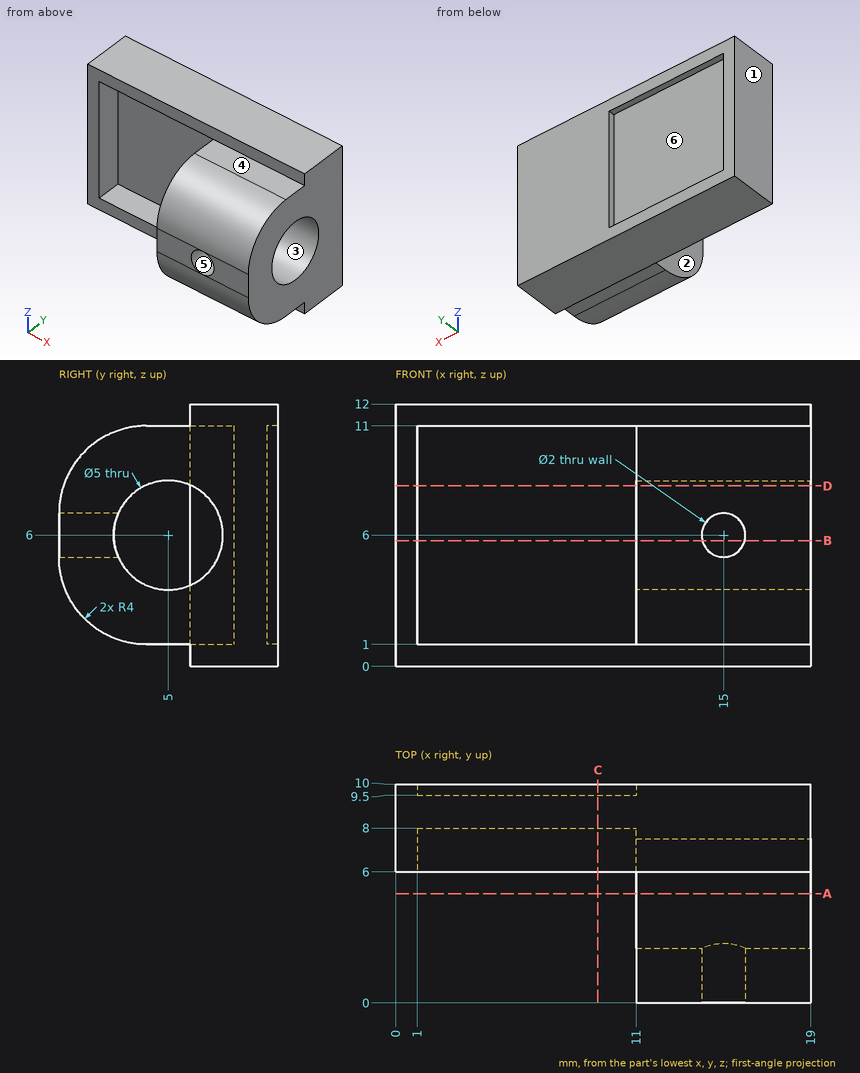
Verification items for this drawing (mm, ordinates from the low corner). A direction names the side the tool comes from. Give positions to 0.01 mm unless a question says otherwise; leave off trailing zeros. Write each loop counter-clockwise with the first axis right and the second up, starting at its lowest first coordinate (ties: lowest second). Pieces come first, ordered by that corner, then holes. Notation, with made-up numbers: (-22, 79) - (-11, 79) arc R15 cw to (-11, 101) - close; hole circle Ø3 at (78.25, 45.5). An arc over 180 degrees is marked (long way). Answer as CSV lines item,"result". Start each with the question number.
1. Draft check along X on the marked faces 1, 2 and 3. Enter one of: pulls with the +X half, pulls with the -X half, needs draft (parallel to the pull), parting line crosses it, or undercut.
2. Depth check by flat-ended pin: pin 1 (4 mm diameter, centred on y = 4.5, z = 8, fed in from -X); pin 2 (0.6 mm diameter, centred on y = 6.5, z = 6.5, fed in from +X); pin 3 (1 mm diameter, centred on x = 8.5, z = 3, fed in from -Y); pin 4 (2 mm diameter, centred on x = 16, y = 4.5, fed in from -Z). Enter the tip coordinate at first touch or a pass-through.
3. Thickness scan on line 1 (Y direction, x = 17, z = 6); line 2 (X direction, y = 1.65, z = 6); line 3 (Y direction, x = 15.5, z = 6). Record the ranges inside material, lowest first.
4. Set-up check for the marked faces 4, 5 and 6: record each of +Z, -Z, +X, -X, +Y, -Y from which the full face is reachable in a straight line by a thin tool's end or side.
5. Sectioned sample at C-C (x = 9.25). Record the boundary of the cut face in (y, z).
6. Sectioned sample at D-D (z = 8.25). Record the boundary of the cut face in (x, y).
7. Sectioned sample at B-B (z = 5.75). Record the boundary of the cut face in (x, y), then the cut area to 3 significant figures.
8. Sectioned sample at A-A (y = 5). Record the boundary of the cut face in (x, z).
Derived:
1,face 1,"pulls with the -X half"
1,face 2,"undercut"
1,face 3,"needs draft"
2,pin 1,"x = 0"
2,pin 2,"x = 1"
2,pin 3,"y = 8"
2,pin 4,"z = 1"
3,line 1,"0 to 2.5, 7.5 to 10"
3,line 2,"11 to 14, 16 to 19"
3,line 3,"7.5 to 10"
4,face 4,"+Z, +X, -X, -Y"
4,face 5,"-Y"
4,face 6,"+Y"
5,outline,"(6, 0) - (10, 0) - (10, 1) - (9.5, 1) - (9.5, 11) - (10, 11) - (10, 12) - (6, 12) - (6, 11) - (8, 11) - (8, 1) - (6, 1) - close"
6,outline,"(0, 6) - (1, 6) - (1, 8) - (11, 8) - (11, 6.09) - (19, 6.09) - (19, 10) - (11, 10) - (11, 9.5) - (1, 9.5) - (1, 10) - (0, 10) - close; (11, 0.2) - (19, 0.2) - (19, 3.91) - (11, 3.91) - close"
7,outline,"(0, 6) - (1, 6) - (1, 8) - (11, 8) - (11, 7.49) - (19, 7.49) - (19, 10) - (11, 10) - (11, 9.5) - (1, 9.5) - (1, 10) - (0, 10) - close; (11, 0) - (14.03, 0) - (14.03, 2.51) - (11, 2.51) - close; (15.97, 0) - (19, 0) - (19, 2.51) - (15.97, 2.51) - close"
7,area,"54.3 mm²"
8,outline,"(11, 1) - (19, 1) - (19, 3.5) - (11, 3.5) - close; (11, 8.5) - (19, 8.5) - (19, 11) - (11, 11) - close"
